Geometry: final body of the model. Coordinates: model frame, mm. Face numbers are marked on the shaded views. A direction names the side the tool comes from. Give positions to 0.01 mm unless a question says otherwise; leave off trailing zeros. Loops run counter-clockwise (first coordinate to the right, second up) from the corner with the lowest first, then second, coordinate; pieces in that order, holes last.
1. Section A-A, the plane y = 14. Output: boundary loops of the cut face in (x, z), then the cut area to 3 significant figures.
2. Material intervals for line 1 along X through (y, z) = (8.25, 5); line 2 along Z through (x, y) = (-14.5, 8.5); line 3 along X through (y, z) = (7.75, -1), sorted ascending.
3. Access query for the marked faces 1, 2 and 3. Directions: +Z, -Z, +X, -X, +Y, -Y. A direction counts if a zero-diameter tool reaches every point of the face in a straight line with its end or side. Return the directions, or none.
4. First-contact query: P1, Ø5, axis at x = 12, y = 12, coming from the +Z side; P2, Ø10, axis at x = 24.5, z = 15, coming from the +Y side; P3, Ø6.5, axis at x = -25, z = -5, coming from the +Y side; P4, Ø1, axis at x = -7.5, y = 14.5, coming from the -Z side. Flat tips, straight axial feed; report the tip coordinate or a pass-through.
5. Section B-B, the plane x = 6. Output: boundary loops of the cut face in (y, z), then the cut area to 3 significant figures.
6. Section C-C, the plane y = 3.75. State how many separate pieces and enclosed holes the cut face has, then the cut area to 3 significant figures.
7. Section D-D, the plane z = 5. Output: boundary loops of the cut face in (x, y), then the cut area to 3 significant figures.
8. Draft query along Z for the marked faces 4, 5 and 6. Return one class per face: +Z half, -Z half, draft (parallel to the pull), parting line (faces both ways), or undercut.
from build123d import *

# Parameters (mm, degrees)
SKETCH_1_W          = 62
SKETCH_1_H          = 25
EXTRUDE_1_DEPTH     = 20
SHELL_1_T           = -2
SKETCH_2_W          = 8
SKETCH_2_H          = 21
EXTRUDE_2_DEPTH     = 8
SKETCH_3_R          = 2
CUT_EXTRUDE_1_DEPTH = 35.889110049
SKETCH_4_R          = 6
CUT_EXTRUDE_2_DEPTH = 38.963798545
SKETCH_5_R          = 2
EXTRUDE_3_DEPTH     = 6
FILLET_1_R          = 4
FILLET_2_R          = 1


with BuildPart() as part:
    # 草图1 → 凸台-拉伸1 (new body)
    with BuildSketch(Plane(origin=(0, 0, 0), x_dir=(1, 0, 0), z_dir=(0, 1, 0))):
        Rectangle(SKETCH_1_W, SKETCH_1_H)
    extrude(amount=EXTRUDE_1_DEPTH)

    # 抽壳1
    shell_1_openings = [part.faces().sort_by_distance(p)[0] for p in [
        (0, 20, 0),
    ]]
    offset(amount=SHELL_1_T, openings=shell_1_openings, kind=Kind.INTERSECTION)

    # 草图2 → 凸台-拉伸2 (add)
    with BuildSketch(Plane(origin=(0, 2, 0), x_dir=(1, 0, 0), z_dir=(0, 1, 0))):
        with Locations((-25, 0)):
            Rectangle(SKETCH_2_W, SKETCH_2_H)
        with Locations((25, 0)):
            Rectangle(SKETCH_2_W, SKETCH_2_H)
    extrude(amount=EXTRUDE_2_DEPTH)

    # 草图3 → 切除-拉伸1 (cut, through all)
    with BuildSketch(Plane(origin=(0, 10, 0), x_dir=(1, 0, 0), z_dir=(0, 1, 0))):
        with Locations(Location((-25, 5, 0), (0, 0, 270))):
            Circle(SKETCH_3_R)
        with Locations(Location((-25, -5, 0), (0, 0, 270))):
            Circle(SKETCH_3_R)
        with Locations(Location((25, 5, 0), (0, 0, 270))):
            Circle(SKETCH_3_R)
        with Locations(Location((25, -5, 0), (0, 0, 270))):
            Circle(SKETCH_3_R)
    extrude(amount=-CUT_EXTRUDE_1_DEPTH, mode=Mode.SUBTRACT)

    # 草图4 → 切除-拉伸2 (cut, through all)
    with BuildSketch(Plane(origin=(0, 2, 0), x_dir=(1, 0, 0), z_dir=(0, 1, 0))):
        with Locations(Location((-12, 0, 0), (0, 0, 270))):
            Circle(SKETCH_4_R)
    extrude(amount=-CUT_EXTRUDE_2_DEPTH, mode=Mode.SUBTRACT)

    # 草图5 → 凸台-拉伸3 (add)
    # profile 1 of 2: a face of its own
    with BuildSketch(Plane(origin=(0, 0, 0), x_dir=(1, 0, 0), z_dir=(0, 1, 0))):
        with BuildLine():
            Line((22.067619242, 18.232380758), (21, 12.5))
            Line((21, 12.5), (31, 12.5))
            Line((31, 12.5), (29.932380758, 18.232380758))
            ThreePointArc((29.932380758, 18.232380758), (26, 21.5), (22.067619242, 18.232380758))
        make_face()
        with Locations(Location((26, 17.5, 0), (0, 0, 270))):
            Circle(SKETCH_5_R, mode=Mode.SUBTRACT)
    # profile 2 of 2: a face of its own
    with BuildSketch(Plane(origin=(0, 0, 0), x_dir=(1, 0, 0), z_dir=(0, 1, 0))):
        with BuildLine():
            Line((2.067619242, 18.232380758), (1, 12.5))
            Line((1, 12.5), (11, 12.5))
            Line((11, 12.5), (9.932380758, 18.232380758))
            ThreePointArc((9.932380758, 18.232380758), (6, 21.5), (2.067619242, 18.232380758))
        make_face()
        with Locations(Location((6, 17.5, 0), (0, 0, 270))):
            Circle(SKETCH_5_R, mode=Mode.SUBTRACT)
    extrude_3 = extrude(amount=EXTRUDE_3_DEPTH)

    # 镜向1: 凸台-拉伸3 across plane
    add(extrude_3.mirror(Plane.XY))

    # 圆角1
    fillet_1_edges = [part.edges().sort_by_distance(p)[0] for p in [
        (-31, 10, 12.5),
        (-31, 10, -12.5),
    ]]
    fillet(fillet_1_edges, radius=FILLET_1_R)

    # 圆角2
    fillet_2_edges = [part.edges().sort_by_distance(p)[0] for p in [
        (29, 15, 10.5),
        (29, 15, -10.5),
        (-29, 15, -10.5),
        (-29, 15, 10.5),
    ]]
    fillet(fillet_2_edges, radius=FILLET_2_R)


solid = part.part
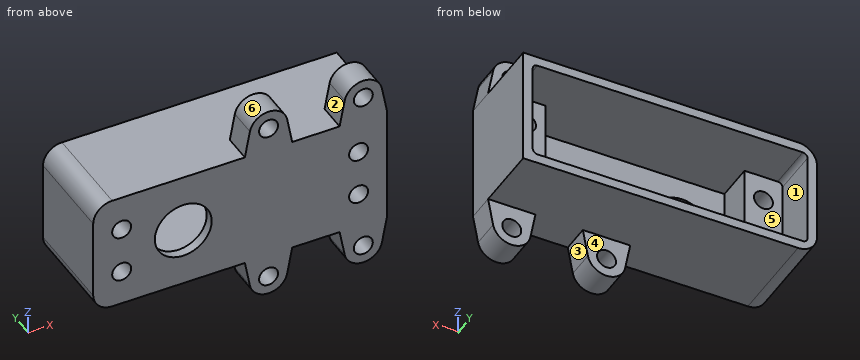
Answers below:
1. outline: (-31, -8.5) arc R4 ccw to (-27, -12.5) - (31, -12.5) - (31, 12.5) - (-27, 12.5) arc R4 ccw to (-31, 8.5) - close; hole (-29, -9.5) arc R1 ccw to (-28, -10.5) - (28, -10.5) arc R1 ccw to (29, -9.5) - (29, 9.5) arc R1 ccw to (28, 10.5) - (-28, 10.5) arc R1 ccw to (-29, 9.5) - close
1. area: 326 mm2
2. line 1: x = -31 to -27, -23 to -21, 21 to 23, 27 to 31
2. line 2: z = -12.5 to -10.5, 10.5 to 12.5
2. line 3: x = -31 to -21, 21 to 31
3. face 1: +Y
3. face 2: +Z, +Y, -Y
3. face 3: -Z, +Y, -Y
4. P1: stops at z = 12.5
4. P2: stops at y = 20
4. P3: stops at y = 10
4. P4: stops at z = -12.5
5. outline: (0, -21.5) - (6, -21.5) - (6, -19.5) - (0, -19.5) - close; (0, -15.5) - (6, -15.5) - (6, -12.5) - (20, -12.5) - (20, -10.5) - (2, -10.5) - (2, 10.5) - (20, 10.5) - (20, 12.5) - (6, 12.5) - (6, 15.5) - (0, 15.5) - close; (0, 19.5) - (6, 19.5) - (6, 21.5) - (0, 21.5) - close
5. area: 182 mm2
6. separate pieces: 1
6. enclosed holes: 9
6. area: 843 mm2
7. outline: (-31, 0) - (-27, 0) - (-27, 10) - (-29, 10) - (-29, 20) - (-31, 20) - close; (-23, 0) - (-15.32, 0) - (-15.32, 2) - (-21, 2) - (-21, 10) - (-23, 10) - close; (-8.68, 0) - (23, 0) - (23, 10) - (21, 10) - (21, 2) - (-8.68, 2) - close; (27, 0) - (31, 0) - (31, 20) - (29, 20) - (29, 10) - (27, 10) - close
7. area: 231 mm2
8. face 4: draft
8. face 5: undercut
8. face 6: +Z half
